The listing builds one solid part. Answer for the finished solid, in the listing's coordinates (mm). Face numbers are marked on the shaded views. A direction names the side the tool comes from. Round coordinates to 2 decimals unless told otherwise and drop trailing zeros. Loops run counter-clockwise (first coordinate to the right, second up) from the corner with the lowest first, then second, coordinate; pieces in that order, holes last. Notation, with made-up numbers: (64, -21.5) -> (108, -21.5) arc R20 cw to (108, -2.5) -> close; hole circle Ø5 at (84, 22). An arc over 180 degrees is marked (long way). One line per question, with ' | ' between items.
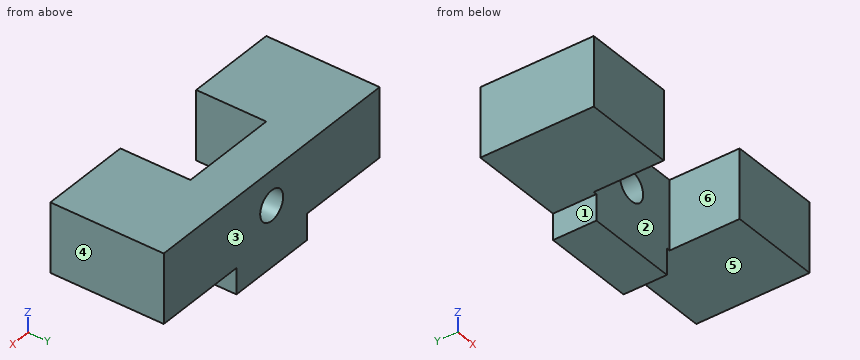
from build123d import *

# Parameters (mm, degrees)
BOSS_EXTRUDE1_DEPTH  = 3.175
SKETCH2_W            = 6.7056
SKETCH2_H            = 5.08
BOSS_EXTRUDE2_DEPTH  = 5.1308
M2_CLEARANCE_HOLE1_D = 2.2


with BuildPart() as part:
    # Sketch1 → Boss-Extrude1 (new body)
    with BuildSketch(Plane(origin=(0, 0, 0), x_dir=(1, 0, 0), z_dir=(0, 1, 0))):
        Polygon((0, 0), (20.6756, 0), (20.6756, 5.08), (13.716, 5.08), (13.716, 6.985), (6.9596, 6.985), (6.9596, 5.08), (0, 5.08), align=None)
    extrude(amount=BOSS_EXTRUDE1_DEPTH)

    # Sketch2 → Boss-Extrude2 (add)
    with BuildSketch(Plane.XZ):
        with Locations((17.3228, -2.54)):
            Rectangle(SKETCH2_W, SKETCH2_H)
        with Locations((3.3528, -2.54)):
            Rectangle(SKETCH2_W, SKETCH2_H)
    extrude(amount=BOSS_EXTRUDE2_DEPTH)

    # M2 Clearance Hole1 (through all)
    with Locations(Plane(origin=(0, 3.175, 0), x_dir=(1, 0, 0), z_dir=(0, 1, 0))):
        with Locations((10.3378, 2.54)):
            Hole(M2_CLEARANCE_HOLE1_D / 2)


solid = part.part
Q1. A cutting plane is placed at B-B on y = -1.75. Give the vertices of the cut face in (x, z), plus the area to 3 significant figures.
Numbers:
outline: (0, -5.08) -> (6.71, -5.08) -> (6.71, 0) -> (0, 0) -> close; (13.97, -5.08) -> (20.68, -5.08) -> (20.68, 0) -> (13.97, 0) -> close | area: 68.1 mm^2
Q2. For the marked faces 1, 2 and 3, determine the directions among +Z, -Z, +X, -X, +Y, -Y from which every point of the face is accessible in a straight line to the end or side of a thin tool.
Numbers:
face 1: -Z, -X, +Y, -Y | face 2: +Z, -Z, -Y | face 3: +Z, -Z, +X, -X, +Y
Q3. Find the intervals of material crossed by line 1 (X direction, y = -3.5, z = -0.75); line 2 (Z direction, x = 18.25, y = -2.5); line 3 (Z direction, x = 10.5, y = 2.75) (3 decimals), in increasing order. Write a range as from..to.
Numbers:
line 1: 0..6.71, 13.97..20.68 | line 2: -5.08..0 | line 3: -6.985..-3.628, -1.452..0
Q4. A cutting plane is placed at D-D on z = -0.75. Give the vertices of the cut face in (x, y) (3 decimals), plus the area to 3 significant figures.
Numbers:
outline: (0, -5.131) -> (6.706, -5.131) -> (6.706, 0) -> (13.97, 0) -> (13.97, -5.131) -> (20.676, -5.131) -> (20.676, 3.175) -> (0, 3.175) -> close | area: 134 mm^2
Q5. A cutting plane is placed at A-A on z = -2.54. Give the vertices of the cut face in (x, y) (3 decimals).
Numbers:
outline: (0, -5.131) -> (6.706, -5.131) -> (6.706, 0) -> (9.238, 0) -> (9.238, 3.175) -> (0, 3.175) -> close; (11.438, 0) -> (13.97, 0) -> (13.97, -5.131) -> (20.676, -5.131) -> (20.676, 3.175) -> (11.438, 3.175) -> close
Q6. A cutting plane is placed at C-C on y = 2. Give the vertices of the cut face in (x, z) (3 decimals), plus the area to 3 significant figures.
Numbers:
outline: (0, -5.08) -> (6.96, -5.08) -> (6.96, -6.985) -> (13.716, -6.985) -> (13.716, -5.08) -> (20.676, -5.08) -> (20.676, 0) -> (0, 0) -> close; hole circle Ø2.2 at (10.338, -2.54) | area: 114 mm^2
Q7. For a pull along X with two mould halves and no side action, classify the marked faces 4, 5 and 6 as pulls with the +X half, pulls with the -X half, needs draft (parallel to the pull), parting line crosses it, or undercut.
Numbers:
face 4: pulls with the +X half | face 5: needs draft | face 6: undercut
Q8. Given pin 1 Ø1.5 at (y, z) = (-2.5, -1.5) entering from -X; pin 2 Ø1 at (y, z) = (1, -6) entering from -X; pin 3 Ø2 at (y, z) = (2.5, -6.5) entering from +X; pin 4 Ø3.5 at (x, z) = (9, -4.5) entering from -Y, each flat-ended and moving along its own axis, determine where each tip first touches the part or whether it passes through.
Numbers:
pin 1: x = 0 | pin 2: x = 6.96 | pin 3: x = 13.72 | pin 4: y = 0
